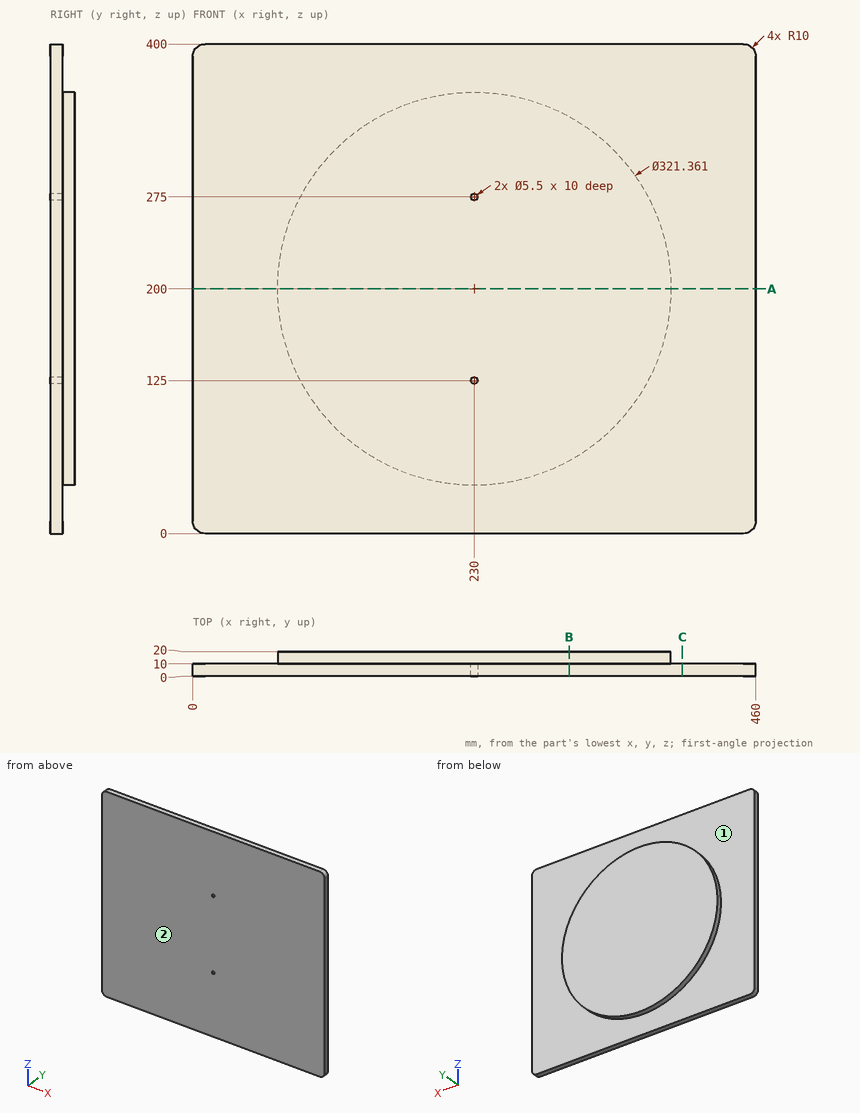
Part print with two shaded views. Sizes in mm from the minimum x, y, z corner. A direction names the side the tool comes from. Round coordinates to 2 decimals unless told otherwise and drop trailing zeros. Loops run counter-clockwise (first coordinate to the right, second up) from the corner with the lowest first, then second, coordinate; pieces in that order, holes last.
Item 1: Saw through at C-C (x = 400). List the corners of the cut face in (y, z), then the cut area to 3 significant figures.
Item 2: Saw through at B-B (x = 307.5). List the corners of the cut face in (y, z), then the cut area to 3 significant figures.
Item 3: Which spindle directions (+Z, -Z, +X, -X, +Y, -Y) get a long thin tool onto all of the face, cutting with end or side? Do the marked faces 1 and 2. Say none if no direction does.
Item 4: Pin check, flat tips, straight feed: P1, Ø1.5, axis at x = 344.5, z = 331, coming from the +Y side; P2, Ø3, axis at y = 17.5, z = 64.5, coming from the +X side; P3, Ø2, axis at y = 13, z = 67.5, coming from the +X side. Stop position of each tip, or through.
Item 5: Saw through at A-A (z = 200). List the corners of the cut face in (x, y), then the cut area to 3 significant figures.
Item 6: Drill centre lines: line 1 along Z through (x, y) = (230, 8.25); line 2 along X through (y, z) = (3.5, 275); line 3 along Y through (x, z) = (197, 40.5). Where is each one in solid material? Low to high.
Worked answers:
1. outline: (0, 0) - (10, 0) - (10, 400) - (0, 400) - close
1. area: 4,000 mm2
2. outline: (0, 0) - (10, 0) - (10, 59.24) - (20, 59.24) - (20, 340.76) - (10, 340.76) - (10, 400) - (0, 400) - close
2. area: 6,820 mm2
3. face 1: +Y
3. face 2: +Z, -Z, +X, -X, -Y
4. P1: stops at y = 10
4. P2: stops at x = 318.67
4. P3: stops at x = 322.34
5. outline: (0, 0) - (460, 0) - (460, 10) - (390.68, 10) - (390.68, 20) - (69.32, 20) - (69.32, 10) - (0, 10) - close
5. area: 7,810 mm2
6. line 1: z = 0 to 122.25, 127.75 to 272.25, 277.75 to 400
6. line 2: x = 0 to 227.25, 232.75 to 460
6. line 3: y = 0 to 10
